from build123d import *

# Parameters (mm, degrees)
SKETCH1_R                           = 5.3975
BOSS_EXTRUDE1_DEPTH                 = 6.35
SKETCH2_R                           = 6.35
CUT_EXTRUDE1_DEPTH                  = 4.7625
SKETCH3_R                           = 6.35
SKETCH3_R_2                         = 5.08
BOSS_EXTRUDE2_DEPTH                 = 4.75996
CHAMFER1_SIZE                       = 0.254
SKETCH4_R                           = 3.81
SKETCH4_R_2                         = 3.175
BOSS_EXTRUDE3_DEPTH                 = 4.75996
CHAMFER2_SIZE                       = 0.254
SKETCH5_R                           = 5.08
SKETCH5_R_2                         = 3.81
BOSS_EXTRUDE4_DEPTH                 = 4.2545
F_6_32_TAPPED_HOLE1_AT_2_COUNT      = 2
F_6_32_TAPPED_HOLE1_AT_2_PITCH      = 26.940768363
F_6_32_TAPPED_HOLE2_D               = 2.7051
F_6_32_TAPPED_HOLE2_DEPTH           = 6.35
F_9_64_0_14063_DIAMETER_HOLE1_D     = 3.572002
F_9_64_0_14063_DIAMETER_HOLE1_DEPTH = 6.35
F_9_64_0_14063_DIAMETER_HOLE1_TIP   = 1.073137666


with BuildPart() as part:
    # Sketch1 → Boss-Extrude1 (new body)
    with BuildSketch(Plane(origin=(0, 0, 0), x_dir=(1, 0, 0), z_dir=(0, 1, 0))):
        with BuildLine():
            Line((-16.764, -16.51), (-7.62, -16.51))
            Line((-7.62, -16.51), (-7.62, -14.9479))
            ThreePointArc((-7.62, -14.9479), (-7.155032015, -13.825367985), (-6.0325, -13.3604))
            Line((-6.0325, -13.3604), (6.0325, -13.3604))
            ThreePointArc((6.0325, -13.3604), (7.155032015, -13.825367985), (7.62, -14.9479))
            Line((7.62, -14.9479), (7.62, -16.51))
            Line((7.62, -16.51), (16.764, -16.51))
            Line((16.764, -16.51), (16.764, -10.4267))
            Line((16.764, -10.4267), (15.1765, -10.4267))
            ThreePointArc((15.1765, -10.4267), (14.053967985, -9.961732015), (13.589, -8.8392))
            Line((13.589, -8.8392), (13.589, 8.8392))
            ThreePointArc((13.589, 8.8392), (14.053967985, 9.961732015), (15.1765, 10.4267))
            Line((15.1765, 10.4267), (16.764, 10.4267))
            Line((16.764, 10.4267), (16.764, 16.51))
            Line((16.764, 16.51), (7.62, 16.51))
            Line((7.62, 16.51), (7.62, 14.9479))
            ThreePointArc((7.62, 14.9479), (7.155032015, 13.825367985), (6.0325, 13.3604))
            Line((6.0325, 13.3604), (-6.0325, 13.3604))
            ThreePointArc((-6.0325, 13.3604), (-7.155032015, 13.825367985), (-7.62, 14.9479))
            Line((-7.62, 14.9479), (-7.62, 16.51))
            Line((-7.62, 16.51), (-16.764, 16.51))
            Line((-16.764, 16.51), (-16.764, 10.4267))
            Line((-16.764, 10.4267), (-15.1765, 10.4267))
            ThreePointArc((-15.1765, 10.4267), (-14.053967985, 9.961732015), (-13.589, 8.8392))
            Line((-13.589, 8.8392), (-13.589, -8.8392))
            ThreePointArc((-13.589, -8.8392), (-14.053967985, -9.961732015), (-15.1765, -10.4267))
            Line((-15.1765, -10.4267), (-16.764, -10.4267))
            Line((-16.764, -10.4267), (-16.764, -16.51))
        make_face()
        Circle(SKETCH1_R, mode=Mode.SUBTRACT)
    extrude(amount=BOSS_EXTRUDE1_DEPTH)

    # Sketch2 → Cut-Extrude1 (cut)
    with BuildSketch(Plane(origin=(0, 6.35, 0), x_dir=(1, 0, 0), z_dir=(0, 1, 0))):
        Circle(SKETCH2_R)
    extrude(amount=-CUT_EXTRUDE1_DEPTH, mode=Mode.SUBTRACT)

    # Sketch3 → Boss-Extrude2 (add)
    with BuildSketch(Plane(origin=(0, 1.5875, 0), x_dir=(-1, 0, 0), z_dir=(0, 1, 0))):
        Circle(SKETCH3_R)
        Circle(SKETCH3_R_2, mode=Mode.SUBTRACT)
    extrude(amount=BOSS_EXTRUDE2_DEPTH)

    # Chamfer1
    chamfer1_edges = [part.edges().sort_by_distance(p)[0] for p in [
        (5.08, 1.5875, 0),
        (5.08, 6.34746, 0),
    ]]
    chamfer(chamfer1_edges, length=CHAMFER1_SIZE)



with BuildPart() as body_2:
    # Sketch4 → Boss-Extrude3 (new body)
    with BuildSketch(Plane(origin=(0, 1.5875, 0), x_dir=(-1, 0, 0), z_dir=(0, 1, 0))):
        Circle(SKETCH4_R)
        Circle(SKETCH4_R_2, mode=Mode.SUBTRACT)
    extrude(amount=BOSS_EXTRUDE3_DEPTH)

    # Chamfer2
    chamfer2_edges = [body_2.edges().sort_by_distance(p)[0] for p in [
        (3.81, 1.5875, 0),
        (3.81, 6.34746, 0),
    ]]
    chamfer(chamfer2_edges, length=CHAMFER2_SIZE)


with BuildPart() as part_1:
    add(part.part)

    add(body_2.part)  # Boss-Extrude4 merges body 2
    # Sketch5 → Boss-Extrude4 (add)
    with BuildSketch(Plane(origin=(0, 6.09346, 0), x_dir=(-1, 0, 0), z_dir=(0, 1, 0))):
        Circle(SKETCH5_R)
        Circle(SKETCH5_R_2, mode=Mode.SUBTRACT)
    extrude(amount=-BOSS_EXTRUDE4_DEPTH)

    # Sketch8 → #6-32 Tapped Hole1 (revolve, cut)
    with BuildSketch(Plane(origin=(-16.764, 3.175, -13.470384182), x_dir=(0, 0, 1), z_dir=(0, 1, 0))):
        Polygon((0, 0), (0, 8.76289403), (1.35255, 7.9502), (1.35255, 7.0104), (1.7526, 7.0104), (1.7526, 0), align=None)
    f_6_32_tapped_hole1 = revolve(axis=Axis((-23.114, 3.175, -13.470384182), (1, 0, 0)), mode=Mode.SUBTRACT)

    # #6-32 Tapped Hole1 at 2: #6-32 Tapped Hole1 ×2
    with Locations(*[(0, 0, i * F_6_32_TAPPED_HOLE1_AT_2_PITCH) for i in range(1, F_6_32_TAPPED_HOLE1_AT_2_COUNT)]):
        add(f_6_32_tapped_hole1, mode=Mode.SUBTRACT)

    # Mirror1: #6-32 Tapped Hole1 across plane
    add(f_6_32_tapped_hole1.mirror(Plane(origin=(0, 0, 0), x_dir=(0, 0, 1), z_dir=(1, 0, 0))), mode=Mode.SUBTRACT)

    # Mirror1 copy 1 sketch → Mirror1 copy 1 (revolve, cut)
    with BuildSketch(Plane(origin=(16.764, 3.175, 13.470384182), x_dir=(0, 0, 1), z_dir=(0, 1, 0))):
        Polygon((0, 0), (0, -8.76289403), (1.35255, -7.9502), (1.35255, -7.0104), (1.7526, -7.0104), (1.7526, 0), align=None)
    revolve(axis=Axis((23.114, 3.175, 13.470384182), (1, 0, 0)), mode=Mode.SUBTRACT)

    # #6-32 Tapped Hole2
    with Locations(Plane(origin=(0, 6.35, 0), x_dir=(-1, 0, 0), z_dir=(0, 1, 0))):
        with Locations((0, -9.525), (-9.525, 0), (0, 9.525), (9.525, 0)):
            Hole(F_6_32_TAPPED_HOLE2_D / 2, depth=F_6_32_TAPPED_HOLE2_DEPTH)

    # 9/64 (0.14063) Diameter Hole1
    with Locations(Plane(origin=(0, 6.35, 0), x_dir=(-1, 0, 0), z_dir=(0, 1, 0))):
        with Locations((6.914797213, -6.914797213), (-6.914797213, -6.914797213), (-6.914797213, 6.914797213), (6.914797213, 6.914797213)):
            Hole(F_9_64_0_14063_DIAMETER_HOLE1_D / 2, depth=F_9_64_0_14063_DIAMETER_HOLE1_DEPTH)
            with Locations((0, 0, -(F_9_64_0_14063_DIAMETER_HOLE1_DEPTH + F_9_64_0_14063_DIAMETER_HOLE1_TIP / 2))):  # 118° drill point
                Cone(0, F_9_64_0_14063_DIAMETER_HOLE1_D / 2, F_9_64_0_14063_DIAMETER_HOLE1_TIP, mode=Mode.SUBTRACT)


solid = part_1.part
Design review of the part built by this model. Coordinates are the model's own, in mm. A direction names the side the tool comes from. Coordinates: 2 decimals unless noted, no trailing zeros. Order: outer loops, then holes, each group sorted by start corner. A loop starts at its lowest first (then second) coordinate and runs counter-clockwise, first axis right, second up.
Item 1: Take a section at B-B, the plane z = 0. Count the separate pieces of the cut face and the enclosed holes in it, then the cut area to 3 significant figures.
Item 2: The part is to be moulded in two halves that separate along Y. For faces 1 (the flat face through (-1, 1.839, 4)), 2 (the cylindrical face through (-7.17, 3.13, 13.84)), 3 (the cylindrical face through (-13.31, 3.1, -15.22)), say which applies: pulls with the +Y half, pulls with the -Y half, needs draft (parallel to the pull), parting line crosses it, or undercut.
Item 3: For faces 4 (the flat face through (-16, 3, -10.427)), 5 (the cylindrical face through (-13.31, 3.1, 11.72)), 6 (the cylindrical face through (-3.978, 0.783, -3.648)), 7 (the flat face through (7.62, 3, 16)), list the 3-axis set-ups (+Z, -Z, +X, -X, +Y, -Y) from which the entire face can be reached by the end or side of a thin tool; tool diameter is ignored.
Item 4: For pin 1 Ø2 at (y, z) = (3.18, -13.47) entering from +X (3 decimals); pin 2 Ø8.5 at (x, z) = (0, 0) entering from +Y; pin 3 Ø1.6 at (x, z) = (-9.525, 0) entering from +Y; pin 4 Ø2 at (y, z) = (3.18, 13.47) entering from -X (3 decimals), all flat-tipped, find the tip position at first contact; note any pin that passes through.
Item 5: Take a section at A-A, the plane x = -13. Write out the cut boundary in (y, z) (3 decimals), then the cut area to 3 significant figures.
Item 6: For line 1 (X direction, y = 4.25, z = -7); line 2 (Z direction, x = 0, y = 1.75) (1 decimal); line 3 (Z direction, x = 13.5, y = 4.75), list the stretches that pass through material, from the lowest coordinate up.
The answers:
1. separate pieces: 4
1. enclosed holes: 0
1. area: 89.3 mm2
2. face 1: pulls with the -Y half
2. face 2: needs draft
2. face 3: undercut
3. face 4: -X, +Y, -Y
3. face 5: -X
3. face 6: -Y
3. face 7: +Z, +Y, -Y
4. pin 1: stops at x = 8.605
4. pin 2: stops at y = 6.35
4. pin 3: passes through
4. pin 4: stops at x = -8.605
5. outline: (0, -16.51) - (6.35, -16.51) - (6.35, 16.51) - (0, 16.51) - close; hole circle Ø3.505 at (3.175, -13.47); hole circle Ø3.505 at (3.175, 13.47)
5. area: 190 mm2
6. line 1: x = -13.59 to -8.7, -5.13 to 5.13, 8.7 to 13.59
6. line 2: z = -13.4 to -10.9, -8.2 to -5.2, -3.7 to -3.2, 3.2 to 3.7, 5.2 to 8.2, 10.9 to 13.4
6. line 3: z = -16.51 to -14.24, -12.7 to 12.7, 14.24 to 16.51
